Here's how the part is built. I have some questions about the finished solid (model axes, mm). Round coordinates to 2 decimals unless told otherwise and drop trailing zeros. Loops run counter-clockwise (first coordinate to the right, second up) from the corner with the lowest first, then second, coordinate; pieces in that order, holes last. Notation, with made-up numbers: (-31, 39) - (27, 39) arc R13 cw to (27, 47) - close; hole circle Ø10 at (1, -19). An arc over 180 degrees is marked (long way). Answer as a JSON object with one key per item and string values. Group by question number.
1) If we mould it in two halves opening along Y, with no side actions, what happens to faces 1 (the face through (2, -49, 2)), 2 (the face through (-0.59, 4.46, 0.99))? For each: pulls with the +Y half, pulls with the -Y half, needs draft (parallel to the pull), parting line crosses it, or undercut.
2) If I drill on line 1 along X through (y, z) = (-120, 1); line 2 along Y through (x, z) = (15, 1.3); line 3 along Y through (x, z) = (11.5, 0.85), over which ranges is the centre line in solid material (lowest first)? Write a range as [from, to].
3) I want a section at B-B, the plane z = 1.55. Give the number of separate pieces and of enclosed holes in the cut face, then the cut area to 3 significant figures.
4) I want a section at A-A, the plane y = 0. Please give me the cut outline in (x, z), then the cut area to 3 significant figures.
5) Will these pins go through, and if not, where does the flat tip stop? P1, Ø1, axis at y = -45.5, z = 1.5, coming from the -X side; P2, Ø0.6, axis at y = -20.5, z = 1.5, coming from the +X side; P3, Ø0.6, axis at y = 11.5, z = 0.5, coming from the +X side.
from build123d import *

# Parameters (mm, degrees)
SKETCH_1_R      = 4.5
SKETCH_1_R_2    = 1
SKETCH_1_W      = 3
SKETCH_1_H      = 4
EXTRUDE_1_DEPTH = 2


with BuildPart() as part:
    # 草图1 → 凸台-拉伸1 (new body)
    with BuildSketch(Plane.XY):
        with BuildLine():
            Line((6, 6), (4, 6))
            Line((4, 6), (4, 16))
            Line((4, 16), (20.5, 16))
            Line((20.5, 16), (20.5, 18))
            Line((20.5, 18), (23, 18))
            Line((23, 18), (23, 16))
            Line((23, 16), (25, 16))
            Line((25, 16), (25, 24))
            Line((25, 24), (23, 24))
            Line((23, 24), (23, 22))
            Line((23, 22), (20.5, 22))
            Line((20.5, 22), (20.5, 24))
            Line((20.5, 24), (-20.5, 24))
            Line((-20.5, 24), (-20.5, 22))
            Line((-20.5, 22), (-23, 22))
            Line((-23, 22), (-23, 24))
            Line((-23, 24), (-25, 24))
            Line((-25, 24), (-25, 16))
            Line((-25, 16), (-23, 16))
            Line((-23, 16), (-23, 18))
            Line((-23, 18), (-20.5, 18))
            Line((-20.5, 18), (-20.5, 16))
            Line((-20.5, 16), (-4, 16))
            Line((-4, 16), (-4, 6))
            Line((-4, 6), (-6, 6))
            Line((-6, 6), (-6, -6))
            Line((-6, -6), (-4, -6))
            Line((-4, -6), (-4, -16))
            Line((-4, -16), (-9, -16))
            Line((-9, -16), (-9, -24))
            Line((-9, -24), (-4, -24))
            Line((-4, -24), (-4, -41))
            Line((-4, -41), (-9, -41))
            Line((-9, -41), (-9, -49))
            Line((-9, -49), (-4, -49))
            Line((-4, -49), (-4, -72))
            Line((-4, -72), (-9, -72))
            Line((-9, -72), (-9, -80))
            Line((-9, -80), (-4, -80))
            Line((-4, -80), (-4, -90))
            add(Edge.make_bspline(
                [(-4, -90), (-12.824800186, -94.946472906), (-14, -105)],
                knots=[0, 0, 0, 1, 1, 1], degree=2))
            Line((-14, -105), (-14, -135))
            Line((-14, -135), (-9, -135))
            Line((-9, -135), (-9, -105.307652325))
            add(Edge.make_bspline(
                [(-1.555258324, -94.361563726), (-4.124118351, -95.824075576), (-6.772437427, -98.85168045), (-8.60156745, -102.414074006), (-9, -105.307652325)],
                knots=[0, 0, 0, 0.368595186, 0.61432531, 0.982920497, 0.982920497, 0.982920497], degree=2))
            add(Edge.make_bspline(
                [(-1.555258324, -94.361563726), (0, -93.652312688), (1.555258324, -94.361563726)],
                knots=[0, 0, 0, 1, 1, 1], degree=2))
            add(Edge.make_bspline(
                [(1.555258324, -94.361563726), (4.124118351, -95.824075576), (6.772437427, -98.85168045), (8.60156745, -102.414074006), (9, -105.307652325)],
                knots=[0, 0, 0, 0.368595186, 0.61432531, 0.982920497, 0.982920497, 0.982920497], degree=2))
            Line((9, -105.307652325), (9, -135))
            Line((9, -135), (14, -135))
            Line((14, -135), (14, -105))
            add(Edge.make_bspline(
                [(4, -90), (12.824800186, -94.946472906), (14, -105)],
                knots=[0, 0, 0, 1, 1, 1], degree=2))
            Line((4, -90), (4, -80))
            Line((4, -80), (9, -80))
            Line((9, -80), (9, -72))
            Line((9, -72), (4, -72))
            Line((4, -72), (4, -49))
            Line((4, -49), (9, -49))
            Line((9, -49), (9, -41))
            Line((9, -41), (4, -41))
            Line((4, -41), (4, -24))
            Line((4, -24), (9, -24))
            Line((9, -24), (9, -16))
            Line((9, -16), (4, -16))
            Line((4, -16), (4, -6))
            Line((4, -6), (6, -6))
            Line((6, -6), (6, 6))
        make_face()
        Circle(SKETCH_1_R, mode=Mode.SUBTRACT)
        with Locations((15, 20.000000004)):
            Circle(SKETCH_1_R_2, mode=Mode.SUBTRACT)
        with Locations((-15, 20.000000004)):
            Circle(SKETCH_1_R_2, mode=Mode.SUBTRACT)
        with Locations((-10, 20.000000004)):
            Circle(SKETCH_1_R_2, mode=Mode.SUBTRACT)
        with Locations((-5, 20.000000004)):
            Circle(SKETCH_1_R_2, mode=Mode.SUBTRACT)
        with Locations((0, 14.54049212)):
            Circle(SKETCH_1_R_2, mode=Mode.SUBTRACT)
        with Locations((0, 9.54049212)):
            Circle(SKETCH_1_R_2, mode=Mode.SUBTRACT)
        with Locations((0, 20.000000004)):
            Circle(SKETCH_1_R_2, mode=Mode.SUBTRACT)
        with Locations((5, 20.000000004)):
            Circle(SKETCH_1_R_2, mode=Mode.SUBTRACT)
        with Locations((10, 20.000000004)):
            Circle(SKETCH_1_R_2, mode=Mode.SUBTRACT)
        with Locations((6, -20)):
            Rectangle(SKETCH_1_W, SKETCH_1_H, mode=Mode.SUBTRACT)
        with Locations((-11.5, -130)):
            Circle(SKETCH_1_R_2, mode=Mode.SUBTRACT)
        with Locations((-11.5, -125)):
            Circle(SKETCH_1_R_2, mode=Mode.SUBTRACT)
        with Locations((-11.5, -120)):
            Circle(SKETCH_1_R_2, mode=Mode.SUBTRACT)
        with Locations((-11.5, -115)):
            Circle(SKETCH_1_R_2, mode=Mode.SUBTRACT)
        with Locations((-6, -76)):
            Rectangle(SKETCH_1_W, SKETCH_1_H, mode=Mode.SUBTRACT)
        with Locations((11.5, -130)):
            Circle(SKETCH_1_R_2, mode=Mode.SUBTRACT)
        with Locations((11.5, -125)):
            Circle(SKETCH_1_R_2, mode=Mode.SUBTRACT)
        with Locations((11.5, -120)):
            Circle(SKETCH_1_R_2, mode=Mode.SUBTRACT)
        with Locations((11.5, -115)):
            Circle(SKETCH_1_R_2, mode=Mode.SUBTRACT)
        Polygon((-3.2, -89.2), (0, -88.2), (3.2, -89.2), (0, -90.2), align=None, mode=Mode.SUBTRACT)
        Polygon((-3.2, -85.2), (0, -84.2), (3.2, -85.2), (0, -86.2), align=None, mode=Mode.SUBTRACT)
        Polygon((-3.2, -81.2), (0, -80.2), (3.2, -81.2), (0, -82.2), align=None, mode=Mode.SUBTRACT)
        with Locations((6, -76)):
            Rectangle(SKETCH_1_W, SKETCH_1_H, mode=Mode.SUBTRACT)
        with Locations((0, -76)):
            Circle(SKETCH_1_R_2, mode=Mode.SUBTRACT)
        Polygon((-3.2, -70.7), (0, -69.7), (3.2, -70.7), (0, -71.7), align=None, mode=Mode.SUBTRACT)
        Polygon((-3.2, -66.7), (0, -65.7), (3.2, -66.7), (0, -67.7), align=None, mode=Mode.SUBTRACT)
        Polygon((-3.2, -62.7), (0, -61.7), (3.2, -62.7), (0, -63.7), align=None, mode=Mode.SUBTRACT)
        Polygon((-3.2, -58.7), (0, -57.7), (3.2, -58.7), (0, -59.7), align=None, mode=Mode.SUBTRACT)
        with Locations((-6, -45)):
            Rectangle(SKETCH_1_W, SKETCH_1_H, mode=Mode.SUBTRACT)
        Polygon((-3.2, -39.2), (0, -38.2), (3.2, -39.2), (0, -40.2), align=None, mode=Mode.SUBTRACT)
        Polygon((-3.2, -34.7), (0, -33.7), (3.2, -34.7), (0, -35.7), align=None, mode=Mode.SUBTRACT)
        Polygon((-3.2, -30.2), (0, -29.2), (3.2, -30.2), (0, -31.2), align=None, mode=Mode.SUBTRACT)
        Polygon((-3.2, -25.7), (0, -24.7), (3.2, -25.7), (0, -26.7), align=None, mode=Mode.SUBTRACT)
        with Locations((-6, -20)):
            Rectangle(SKETCH_1_W, SKETCH_1_H, mode=Mode.SUBTRACT)
        with Locations((0, -15)):
            Circle(SKETCH_1_R_2, mode=Mode.SUBTRACT)
        with Locations((0, -10)):
            Circle(SKETCH_1_R_2, mode=Mode.SUBTRACT)
        Polygon((-3.2, -54.7), (0, -53.7), (3.2, -54.7), (0, -55.7), align=None, mode=Mode.SUBTRACT)
        Polygon((-3.2, -50.7), (0, -49.7), (3.2, -50.7), (0, -51.7), align=None, mode=Mode.SUBTRACT)
        with Locations((0, -45)):
            Circle(SKETCH_1_R_2, mode=Mode.SUBTRACT)
        with Locations((6, -45)):
            Rectangle(SKETCH_1_W, SKETCH_1_H, mode=Mode.SUBTRACT)
        with Locations((0, -20)):
            Circle(SKETCH_1_R_2, mode=Mode.SUBTRACT)
    extrude(amount=EXTRUDE_1_DEPTH)


solid = part.part
Outcome:
{
 "1": {"face 1": "needs draft", "face 2": "undercut"},
 "2": {"line 1": "[-14, -12.5], [-10.5, -9], [9, 10.5], [12.5, 14]", "line 2": "[16, 19], [21, 24]", "line 3": "[-135, -131], [-129, -126], [-124, -121], [-119, -116], [-114, -97.17], [16, 24]"},
 "3": {"separate pieces": "1", "enclosed holes": "42", "area": "1,710 mm^2"},
 "4": {"outline": "(-6, 0) - (-4.5, 0) - (-4.5, 2) - (-6, 2) - close; (4.5, 0) - (6, 0) - (6, 2) - (4.5, 2) - close", "area": "6.00 mm^2"},
 "5": {"P1": "x = -9", "P2": "x = 9", "P3": "x = 4"}
}
